Geometry check sheet. Reference: the model listing, model coordinates, mm. Face numbers are marked on the shaded views. A direction names the side the tool comes from. Round coordinates to 2 decimals unless told otherwise and drop trailing zeros. Loops run counter-clockwise (first coordinate to the right, second up) from the corner with the lowest first, then second, coordinate; pieces in that order, holes last. Notation, with made-up numbers: (76, 52) - (113, 52) arc R24 cw to (113, 67) - close; hole circle Ø9 at (29, -39.75). An arc over 180 degrees is marked (long way). Write item = value, one per line.
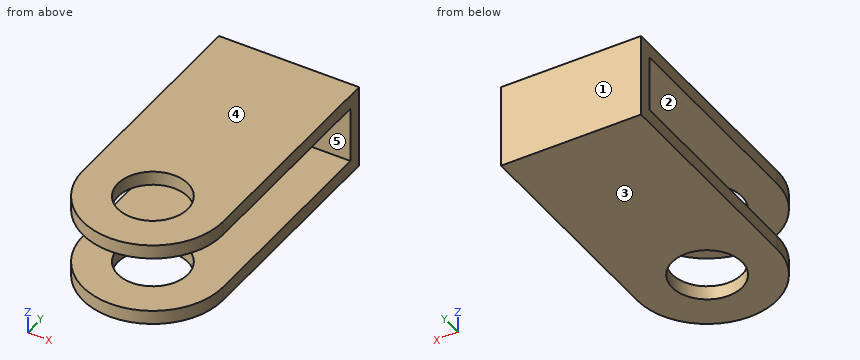
```python
from build123d import *

# Parameters (mm, degrees)
SKETCH1_R           = 5
BOSS_EXTRUDE1_DEPTH = 12
CUT_EXTRUDE1_REACH  = 52.006
SKETCH2_W           = 8
SKETCH2_H           = 42.233489427


with BuildPart() as part:
    # Sketch1 → Boss-Extrude1 (new body)
    with BuildSketch(Plane.XY):
        with BuildLine():
            Line((-2.088637096, 12.233489427), (-2.088637096, 44.233489427))
            Line((-2.088637096, 44.233489427), (17.911362904, 44.233489427))
            Line((17.911362904, 44.233489427), (17.911362904, 12.233489427))
            ThreePointArc((17.911362904, 12.233489427), (7.911362904, 2.233489427), (-2.088637096, 12.233489427))
        make_face()
        with Locations((7.911362904, 12.233489427)):
            Circle(SKETCH1_R, mode=Mode.SUBTRACT)
    extrude(amount=BOSS_EXTRUDE1_DEPTH)

    # Cut-Extrude1: up to this face of the body (flat: up to its plane)
    cut_extrude1_end = Plane(part.part.faces().sort_by_distance((17.911362904, 28.233489427, 6))[0])
    # Sketch2 → Cut-Extrude1 (cut, up to the picked face)
    with BuildSketch(Plane.ZY.offset(2.088637096), mode=Mode.PRIVATE) as cut_extrude1_sk1:
        with Locations((6, 21.116744714)):
            Rectangle(SKETCH2_W, SKETCH2_H)
    cut_extrude1_tool1 = split(extrude(cut_extrude1_sk1.sketch, amount=-CUT_EXTRUDE1_REACH, mode=Mode.PRIVATE), bisect_by=cut_extrude1_end, keep=Keep.BOTH, mode=Mode.PRIVATE)
    add(cut_extrude1_tool1.solids().sort_by(Axis((-2.088637, 21.116745, 6), (1, 0, 0)))[0], mode=Mode.SUBTRACT)


solid = part.part
```
(1) Gauge pin test, flat ends, axial feed: pin 1 (5 mm diameter, centred on x = 5, y = 28, fed in from -Z); pin 2 (6 mm diameter, centred on x = 6.5, z = 5.5, fed in from -Y). Record the tip position at first contact, or that the pin passes through.
Answers follow:
pin_1 = 0
pin_2 = 42.23
(2) Scan lines: L1, parallel to Z at x = 15.75, y = 8; L2, parallel to X at y = 8, z = 11; L3, parallel to Y at x = 12, z = 8.75. Record each from-to range of solid material in increasing order. Write a range as [from, to].
Answers follow:
L1 = [0, 2], [10, 12]
L2 = [-1.15, 5.25], [10.57, 16.97]
L3 = [42.23, 44.23]
(3) Section check D-D (z = 6.5). Enter the section's corners in (x, y), then the cut area to 3 significant figures.
Answers follow:
outline = (-2.09, 42.23) - (17.91, 42.23) - (17.91, 44.23) - (-2.09, 44.23) - close
area = 40.0 mm²
(4) Section check A-A (y = 40). Enter the section's corners in (x, z), then the cut area to 3 significant figures.
Answers follow:
outline = (-2.09, 0) - (17.91, 0) - (17.91, 2) - (-2.09, 2) - close; (-2.09, 10) - (17.91, 10) - (17.91, 12) - (-2.09, 12) - close
area = 80.0 mm²
(5) Mould release check, pull along Z, two halves, no side actions. Record for the marked faces 3, 4 and 5: pulls with the +Z half, pulls with the -Z half, needs draft (parallel to the pull), parting line crosses it, or undercut.
Answers follow:
face_3 = pulls with the -Z half
face_4 = pulls with the +Z half
face_5 = undercut
(6) Section check C-C (z = 11). Enter the section's corners in (x, y).
Answers follow:
outline = (-2.09, 12.23) arc R10 ccw to (17.91, 12.23) - (17.91, 44.23) - (-2.09, 44.23) - close; hole circle Ø10 at (7.91, 12.23)
(7) Section check B-B (x = 5). Enter the section's corners in (y, z).
Answers follow:
outline = (2.67, 0) - (8.17, 0) - (8.17, 2) - (2.67, 2) - close; (2.67, 10) - (8.17, 10) - (8.17, 12) - (2.67, 12) - close; (16.3, 0) - (44.23, 0) - (44.23, 12) - (16.3, 12) - (16.3, 10) - (42.23, 10) - (42.23, 2) - (16.3, 2) - close
(8) Set-up check for the marked faces 1 and 2: record each of +Z, -Z, +X, -X, +Y, -Y from which the full face is reachable in a straight line by a thin tool's end or side.
Answers follow:
face_1 = +Z, -Z, +X, -X, +Y
face_2 = +X, -X, -Y
